The model under review builds one solid part; all positions refer to its coordinate system, in mm. Give positions to 0.01 mm unless a question says otherwise; leave off trailing zeros. Loops run counter-clockwise (first coordinate to the right, second up) from the corner with the lowest first, then second, coordinate; pieces in that order, holes last. Notation, with made-up numbers: (89.5, 82) - (93.5, 82) arc R21 cw to (93.5, 118) - close; hole circle Ø7 at (24.25, -15.75). An arc over 180 degrees is marked (long way). Answer as a JSON object with one key per item and string values.
from build123d import *

# Parameters (mm, degrees)
SKETCH1_W           = 90
SKETCH1_H           = 155.172413794
SKETCH1_R           = 1.655172414
BOSS_EXTRUDE1_DEPTH = 3
CUT_EXTRUDE1_DEPTH  = 90.741960646
CHAMFER1_SIZE       = 1
CHAMFER2_SIZE       = 1
SKETCH6_R           = 2
CUT_EXTRUDE2_DEPTH  = 3


with BuildPart() as part:
    # Sketch1 → Boss-Extrude1 (new body)
    with BuildSketch(Plane(origin=(0, 0, 0), x_dir=(1, 0, 0), z_dir=(0, 1, 0))):
        Rectangle(SKETCH1_W, SKETCH1_H)
        with Locations(Location((38.5, -70, 0), (0, 0, 270))):
            Circle(SKETCH1_R, mode=Mode.SUBTRACT)
        with Locations(Location((-38.5, -70, 0), (0, 0, 270))):
            Circle(SKETCH1_R, mode=Mode.SUBTRACT)
        with Locations(Location((38.5, 70, 0), (0, 0, 270))):
            Circle(SKETCH1_R, mode=Mode.SUBTRACT)
        with Locations(Location((-38.5, 70, 0), (0, 0, 270))):
            Circle(SKETCH1_R, mode=Mode.SUBTRACT)
    extrude(amount=BOSS_EXTRUDE1_DEPTH)

    # Sketch2 → Cut-Extrude1 (cut, through all)
    with BuildSketch(Plane(origin=(0, 3, 0), x_dir=(1, 0, 0), z_dir=(0, 1, 0))):
        with BuildLine():
            ThreePointArc((-39.9, 46.5), (-42.63137085, 47.63137085), (-41.5, 44.9))
            Line((-41.5, 44.9), (-41.5, 46.5))
            Line((-41.5, 46.5), (-39.9, 46.5))
        make_face()
        with BuildLine():
            Line((-41.5, 46.5), (-41.5, 44.9))
            ThreePointArc((-41.5, 44.9), (-40.36862915, 45.36862915), (-39.9, 46.5))
            Line((-39.9, 46.5), (-41.5, 46.5))
        make_face()
        with BuildLine():
            ThreePointArc((39.9, 46.5), (40.36862915, 45.36862915), (41.5, 44.9))
            Line((41.5, 44.9), (41.5, 46.5))
            Line((41.5, 46.5), (39.9, 46.5))
        make_face()
        with BuildLine():
            Line((41.5, 46.5), (41.5, 44.9))
            ThreePointArc((41.5, 44.9), (42.63137085, 45.36862915), (43.1, 46.5))
            ThreePointArc((43.1, 46.5), (41.5, 48.1), (39.9, 46.5))
            Line((39.9, 46.5), (41.5, 46.5))
        make_face()
        with BuildLine():
            ThreePointArc((41.5, -44.9), (40.36862915, -45.36862915), (39.9, -46.5))
            Line((39.9, -46.5), (41.5, -46.5))
            Line((41.5, -46.5), (41.5, -44.9))
        make_face()
        with BuildLine():
            Line((41.5, -46.5), (39.9, -46.5))
            ThreePointArc((39.9, -46.5), (41.5, -48.1), (43.1, -46.5))
            ThreePointArc((43.1, -46.5), (42.63137085, -45.36862915), (41.5, -44.9))
            Line((41.5, -44.9), (41.5, -46.5))
        make_face()
        with BuildLine():
            Line((-41.5, -44.9), (-41.5, -46.5))
            Line((-41.5, -46.5), (-39.9, -46.5))
            ThreePointArc((-39.9, -46.5), (-40.36862915, -45.36862915), (-41.5, -44.9))
        make_face()
        with BuildLine():
            Line((-39.9, -46.5), (-41.5, -46.5))
            Line((-41.5, -46.5), (-41.5, -44.9))
            ThreePointArc((-41.5, -44.9), (-42.63137085, -47.63137085), (-39.9, -46.5))
        make_face()
    extrude(amount=-CUT_EXTRUDE1_DEPTH, mode=Mode.SUBTRACT)

    # Chamfer1
    chamfer1_edges = [part.edges().sort_by_distance(p)[0] for p in [
        (0, 3, 77.586206897),
        (0, 3, -77.586206897),
    ]]
    chamfer(chamfer1_edges, length=CHAMFER1_SIZE)

    # Chamfer2
    chamfer2_edges = [part.edges().sort_by_distance(p)[0] for p in [
        (45, 3, 0),
        (-45, 3, 0),
    ]]
    chamfer(chamfer2_edges, length=CHAMFER2_SIZE)

    # Sketch6 → Cut-Extrude2 (cut)
    with BuildSketch(Plane(origin=(0, 3, 0), x_dir=(1, 0, 0), z_dir=(0, 1, 0))):
        with Locations(Location((15, -59.586206897, 0), (0, 0, 270))):
            Circle(SKETCH6_R)
        with Locations(Location((15, 59.586206897, 0), (0, 0, 270))):
            Circle(SKETCH6_R)
    extrude(amount=-CUT_EXTRUDE2_DEPTH, mode=Mode.SUBTRACT)


solid = part.part
Q1. Clearance check with a flat-ended pin moving along its axis: pin 1 Ø5 at (x, z) = (15, 59.59) entering from +Y. State where the tip first meets the part, or that it passes through.
Results:
{"pin 1": "stops at y = 3"}
Q2. Consider section B-B, the plane z = 70. State the section outline as (x, y) points.
Results:
{"outline": "(-45, 0) - (-40.16, 0) - (-40.16, 3) - (-44, 3) - (-45, 2) - close; (-36.84, 0) - (36.84, 0) - (36.84, 3) - (-36.84, 3) - close; (40.16, 0) - (45, 0) - (45, 2) - (44, 3) - (40.16, 3) - close"}
Q3. The part is to be moulded in two halves that separate along Z. For faces 1 (the face through (-1, 3, -1)), 2 (the face through (37.87, 1.48, 71.53)), say which applies: +Z half, -Z half, draft (parallel to the pull), parting line (faces both ways), or undercut.
Results:
{"face 1": "draft", "face 2": "undercut"}
Q4. To check wall thickness, follow probe 1 along X at (y, z) = (2.1, -46.5); probe 2 along Z at (x, y) = (-41.5, 1.3); probe 3 along X at (y, z) = (1.9, 70). State the ranges of each line that lie inside material, in increasing order. Write a range as [from, to].
Results:
{"probe 1": "x = [-44.9, -43.1], [-39.9, 39.9], [43.1, 44.9]", "probe 2": "z = [-77.59, -48.1], [-44.9, 44.9], [48.1, 77.59]", "probe 3": "x = [-45, -40.16], [-36.84, 36.84], [40.16, 45]"}
Q5. Consider section A-A, the plane x = 15. State the section outline as (y, z) points, plus the area to 3 significant figures.
Results:
{"outline": "(0, -77.59) - (2, -77.59) - (3, -76.59) - (3, -61.59) - (0, -61.59) - close; (0, -57.59) - (3, -57.59) - (3, 57.59) - (0, 57.59) - close; (0, 61.59) - (3, 61.59) - (3, 76.59) - (2, 77.59) - (0, 77.59) - close", "area": "441 mm^2"}
